CAD build for the part. Positions are in the model's coordinates, mm. A direction names the side the tool comes from. Coordinates: 2 decimals unless noted, no trailing zeros. Loops run counter-clockwise (first coordinate to the right, second up) from the corner with the lowest first, then second, coordinate; pieces in that order, holes last.
1) Saw through at B-B, the plane y = 118.5. Write the cut outline in (x, z), and give its area (3 significant figures).
2) Saw through at A-A, the plane x = -14. Write the cut outline in (y, z).
3) Wall check: line 1 along X through (y, z) = (4, 0.9); line 2 along X through (y, z) = (33.5, 3.65); line 3 along Y through (x, z) = (6, 2.85). Give the ranges that are in metal, low to high.
4) Two-plate mould, pull along Y, no slides. Class faces 5 (the cylindrical face through (11.047, 23.611, 2.535)), 6 (the flat face through (-30, 71, 2)), 7 (the flat face through (0, 14, 2)): +Y half, -Y half, draft (parallel to the pull), parting line (faces both ways), or undercut.
5) Which spindle directions (+Z, -Z, +X, -X, +Y, -Y) get a long thin tool onto all of the face, cutting with end or side? Do faces 1 (the flat face through (0, -10, 2)), 2 (the flat face through (-5, 11, 2)), 3 (the flat face through (1, 33, 2)), 4 (the flat face through (2, 28, 2)). Say none if no direction does.
6) Pin check, flat tips, straight feed: pin 1 Ø2.5 at (x, z) = (0, 2) entering from +Y; pin 2 Ø3 at (x, z) = (2, 1.5) entering from -Y; pin 3 Ø2.5 at (y, z) = (13, 2) entering from +X. Stop position of each tip, or through.
```python
from build123d import *

# Parameters (mm, degrees)
EXTRUDE_1_DEPTH     = 5
FILLET_1_R          = 2.5
FILLET_2_R          = 1
EXTRUDE_2_DEPTH     = 8
FILLET_3_R          = 2.5
SKETCH_5_W          = 1.467751534
SKETCH_5_H          = 4.178210798
SKETCH_5_W_2        = 1.389566385
CUT_EXTRUDE_1_DEPTH = 20
FILLET_4_R          = 1.5
FILLET_5_R          = 1.5


with BuildPart() as part:
    # 草图1 → 凸台-拉伸1 (new body)
    with BuildSketch(Plane.XY):
        Polygon((0, 0), (0, 28), (4, 28), (7.380946094, 20.749537704), (11.912485029, 22.862629012), (7.185351304, 33), (-5, 33), (-5, -12), (-30, -12), (-30, 158), (-35, 158), (-35, -17), (0, -17), (0, -5), (8, -5), (8, 0), align=None)
    extrude(amount=EXTRUDE_1_DEPTH)

    # 圆角1
    fillet_1_edges = [part.edges().sort_by_distance(p)[0] for p in [
        (-32.5, 158, 0),
        (9.646715562, 21.806083358, 0),
        (9.646715562, 21.806083358, 5),
        (-35, 158, 2.5),
        (-30, 158, 2.5),
        (7.185351304, 33, 2.5),
        (11.912485029, 22.862629012, 2.5),
        (7.380946094, 20.749537704, 2.5),
        (-32.5, 158, 5),
    ]]
    fillet(fillet_1_edges, radius=FILLET_1_R - 0.0001)  # a hair under: the kernel refuses the full size

    # 圆角2
    fillet_2_edges = [part.edges().sort_by_distance(p)[0] for p in [
        (-5, 33, 2.5),
    ]]
    fillet(fillet_2_edges, radius=FILLET_2_R)

    # 草图3 → 凸台-拉伸2 (add)
    with BuildSketch(Plane(origin=(0, 0, 0), x_dir=(0, 0, -1), z_dir=(1, 0, 0))):
        with BuildLine():
            Line((-5, 0), (0, 0))
            ThreePointArc((0, 0), (-2.5, 2.5), (-5, 0))
        make_face()
    extrude(amount=EXTRUDE_2_DEPTH)

    # 圆角3
    fillet_3_edges = [part.edges().sort_by_distance(p)[0] for p in [
        (8, -2.5, 0),
        (8, -5, 2.5),
        (8, -2.5, 5),
        (8, 2.5, 2.5),
    ]]
    fillet(fillet_3_edges, radius=FILLET_3_R - 0.0001)  # a hair under: the kernel refuses the full size

    # 草图4 → 旋转3 (revolve)
    with BuildSketch(Plane(origin=(4.4, 0, 0), x_dir=(0, 0, -1), z_dir=(1, 0, 0))):
        with BuildLine():
            Line((-5.5, 0), (0.5, 0))
            ThreePointArc((0.5, 0), (-2.5, 3), (-5.5, 0))
        make_face()
    revolve(axis=Axis((4.4, 0, 2.5), (0, 0, -1)))

    # 草图5 → 切除-拉伸1 (cut)
    with BuildSketch(Plane.ZY.offset(5)):
        with Locations((-0.733875767, -0.010051234)):
            Rectangle(SKETCH_5_W, SKETCH_5_H)
        with Locations((5.694783193, -0.010051234)):
            Rectangle(SKETCH_5_W_2, SKETCH_5_H)
    extrude(amount=-CUT_EXTRUDE_1_DEPTH, mode=Mode.SUBTRACT)

    # 圆角4
    fillet_4_edges = [part.edges().sort_by_distance(p)[0] for p in [
        (-30, -12, 2.5),
        (-5, -12, 2.5),
    ]]
    fillet(fillet_4_edges, radius=FILLET_4_R)

    # 圆角5
    fillet_5_edges = [part.edges().sort_by_distance(p)[0] for p in [
        (0, -17, 2.5),
        (-35, -17, 2.5),
    ]]
    fillet(fillet_5_edges, radius=FILLET_5_R)


solid = part.part
```
Data:
1. outline: (-35, 0) - (-30, 0) - (-30, 5) - (-35, 5) - close
1. area: 25.0 mm2
2. outline: (-17, 0) - (-12, 0) - (-12, 5) - (-17, 5) - close
3. line 1: x = -35 to -30, -5 to 0
3. line 2: x = -35 to -30
3. line 3: y = -4.95 to 2.51, 23.71 to 32.97
4. face 5: parting line
4. face 6: draft
4. face 7: undercut
5. face 1: +Z, -Z, +X, -Y
5. face 2: +Z, -Z, +Y
5. face 3: +Z, -Z, +X, +Y
5. face 4: +Z, -Z
6. pin 1: stops at y = 33
6. pin 2: stops at y = -5
6. pin 3: stops at x = 0
